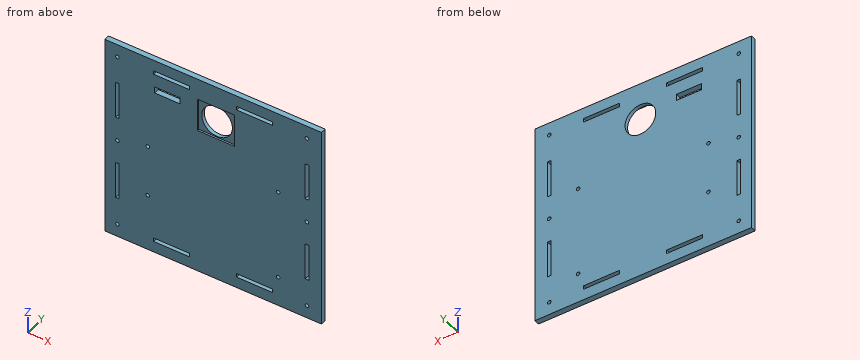
from build123d import *

# Parameters (mm, degrees)
F0_W     = 120
F0_H     = 110
F0_R     = 1
F0_W_2   = 20
F0_H_2   = 2
F0_W_3   = 2
F0_H_3   = 20
F0_W_4   = 14
F0_H_4   = 3.5
F0_R_2   = 8.5
F1_DEPTH = 3
F2_W     = 20.5
F2_H     = 18
F2_R     = 8.5
F3_DEPTH = 1


with BuildPart() as f1:
    # F0 (on Front) → F1 (new body)
    with BuildSketch(Plane.XZ):
        Rectangle(F0_W, F0_H)
        with Locations((-53, -48)):
            Circle(F0_R, mode=Mode.SUBTRACT)
        with Locations((-23, -48)):
            Rectangle(F0_W_2, F0_H_2, mode=Mode.SUBTRACT)
        with Locations((-53, -23)):
            Rectangle(F0_W_3, F0_H_3, mode=Mode.SUBTRACT)
        with Locations((-36.223244, -23.959939)):
            Circle(F0_R, mode=Mode.SUBTRACT)
        with Locations((23, -48)):
            Rectangle(F0_W_2, F0_H_2, mode=Mode.SUBTRACT)
        with Locations((52, -48)):
            Circle(F0_R, mode=Mode.SUBTRACT)
        with Locations((36.031369, -38.8)):
            Circle(F0_R, mode=Mode.SUBTRACT)
        with Locations((52, -23)):
            Rectangle(F0_W_3, F0_H_3, mode=Mode.SUBTRACT)
        with Locations((-53, 0)):
            Circle(F0_R, mode=Mode.SUBTRACT)
        with Locations((-36.223244, 4.040061)):
            Circle(F0_R, mode=Mode.SUBTRACT)
        with Locations((-53, 23)):
            Rectangle(F0_W_3, F0_H_3, mode=Mode.SUBTRACT)
        with Locations((-53, 48)):
            Circle(F0_R, mode=Mode.SUBTRACT)
        with Locations((-25.438215, 38.25)):
            Rectangle(F0_W_4, F0_H_4, mode=Mode.SUBTRACT)
        with Locations((-23, 48)):
            Rectangle(F0_W_2, F0_H_2, mode=Mode.SUBTRACT)
        with Locations((36.031369, 10)):
            Circle(F0_R, mode=Mode.SUBTRACT)
        with Locations((52, 0)):
            Circle(F0_R, mode=Mode.SUBTRACT)
        with Locations((52, 23)):
            Rectangle(F0_W_3, F0_H_3, mode=Mode.SUBTRACT)
        with Locations((1.5, 34.534223)):
            Circle(F0_R_2, mode=Mode.SUBTRACT)
        with Locations((23, 48)):
            Rectangle(F0_W_2, F0_H_2, mode=Mode.SUBTRACT)
        with Locations((52, 48)):
            Circle(F0_R, mode=Mode.SUBTRACT)
    extrude(amount=F1_DEPTH)

    # F2 (on face) → F3 (cut)
    with BuildSketch(Plane.XZ.offset(3)):
        with Locations((1.5, 34.534223)):
            Rectangle(F2_W, F2_H)
        with Locations((1.5, 34.534223)):
            Circle(F2_R, mode=Mode.SUBTRACT)
    extrude(amount=-F3_DEPTH, mode=Mode.SUBTRACT)


solid = f1.part
Can you work these out from the model? Positions are in its coordinate system, mm. Coordinates: 2 decimals unless noted, no trailing zeros. Write each loop counter-clockwise with the first axis right and the second up, starting at its lowest first coordinate (ties: lowest second). Pieces come first, ordered by that corner, then holes. Notation, with made-up numbers: (10.25, -5.75) -> (55.25, -5.75) arc R11 cw to (55.25, 12.25) -> close; hole circle Ø1 at (18.5, -1.5). An arc over 180 degrees is marked (long way). Write each question's results on one line, items separated by ' | '. Start each with the question number.
Item 1: If we section it at A-A, the plane x = 25: Write out the boundary of the cut face in (y, z), and give its area (3 significant figures).
Item 2: If we section it at D-D, the plane y = -1.5: Count the separate pieces of the cut face and the enclosed holes in it, and give its area (3 significant figures).
Item 3: Please list where these lines run through material, in increasing order: probe 1 along Z at (x, y) = (-28, -0.5); probe 2 along X at (y, z) = (-2.75, -16.5); probe 3 along Z at (x, y) = (52, -0.85).
Item 4: If we section it at B-B, the plane x = -29: Write out the boundary of the cut face in (y, z).
Item 5: If we section it at C-C, the plane x = 5.5: Write out the boundary of the cut face in (y, z), and give its area (3 significant figures).
Item 6: I'm going to push a flat-ended pin straight in: P1, Ø6, axis at x = -4.5, z = 38.5, coming from the +Y side. Where does the tip first touch, or does it pass through?
Answer block:
1) outline: (-3, -55) -> (0, -55) -> (0, -49) -> (-3, -49) -> close; (-3, -47) -> (0, -47) -> (0, 47) -> (-3, 47) -> close; (-3, 49) -> (0, 49) -> (0, 55) -> (-3, 55) -> close | area: 318 mm²
2) separate pieces: 1 | enclosed holes: 20 | area: 12,600 mm²
3) probe 1: -55 to -49, -47 to 36.5, 40 to 47, 49 to 55 | probe 2: -60 to -54, -52 to 51, 53 to 60 | probe 3: -55 to -49, -47 to -33, -13 to -1, 1 to 13, 33 to 47, 49 to 55
4) outline: (-3, -55) -> (0, -55) -> (0, -49) -> (-3, -49) -> close; (-3, -47) -> (0, -47) -> (0, 36.5) -> (-3, 36.5) -> close; (-3, 40) -> (0, 40) -> (0, 47) -> (-3, 47) -> close; (-3, 49) -> (0, 49) -> (0, 55) -> (-3, 55) -> close
5) outline: (-3, -55) -> (0, -55) -> (0, 27.03) -> (-2, 27.03) -> (-2, 25.53) -> (-3, 25.53) -> close; (-3, 43.53) -> (-2, 43.53) -> (-2, 42.03) -> (0, 42.03) -> (0, 55) -> (-3, 55) -> close | area: 282 mm²
6) P1: y = 0
